For this review, take the finished solid that the model builds, in its own axes (mm). A direction names the side the tool comes from. Give positions to 0.01 mm unless a question says otherwise; leave off trailing zeros. Write each loop counter-clockwise with the first axis right and the second up, starting at its lowest first coordinate (ties: lowest second). Pieces come first, ordered by that corner, then holes.
Q1. Machinability: for faces 1 (the flat face through (1, 30, -11.75)), 2 (the cylindrical face through (0.57, 19.27, -14.4)), 3 (the cylindrical face through (30.43, 43.48, -14.4)), 4 (the flat face through (27, 19, -7)), 5 (the flat face through (13, 37, -1)), which of the approach directions +Z, -Z, +X, -X, +Y, -Y give a long, thin tool a straight path to every point of the face, cutting with its end or side? Answer none if there is none.
Q2. We need section B-B (y = 22.5). Write out the cut boundary in (x, z).
Q3. We need section C-C (x = 13.5). Write out the cut boundary in (y, z), then the cut area to 4 significant figures.
Q4. For line 1 (X direction, y = 22.5, z = -11.2); line 2 (Y direction, x = 13.5, z = -7); line 3 (X direction, y = 7, z = -11.25), list the stretches that pass through material, from the lowest coordinate up.
Q5. Mouldability with a two-part tool opening along X and no side actions: class faces 6 (the flat face through (9.4, 45, -14.3)), 7 (the cylindrical face through (-3.4, 43.48, -0.57)), 8 (the cylindrical face through (26.43, 19.27, -14.4)), 9 (the flat face through (13, 37, -14)) as released by +X, released by -X, zero draft, split by the parting line, or undercut.
Q6. Insertion check: P1, Ø4, axis at x = 4.5, z = -10.5, coming from the +Y side; P2, Ø2, axis at y = 36, z = -6, coming from the -X side; P3, Ø1.5, axis at y = 29.5, z = -10, coming from the -X side; P4, Ø4.5, axis at x = 13.5, y = 22.5, coming from the -Z side. Each pin has a flat end and moves straight along its axis. Give the tip position at first contact, or say it passes through.
Q7. We need section D-D (y = 36.5). Write out the cut boundary in (x, z).
Q8. We need section A-A (z = -6). Give the number of separate pieces and of enclosed holes in the cut face, then the cut area to 3 significant figures.
```python
from build123d import *

# Parameters (mm, degrees)
SKETCH1_W           = 27
SKETCH1_H           = 15
BOSS_EXTRUDE1_DEPTH = 45
SKETCH2_W           = 35
SKETCH2_H           = 15
BOSS_EXTRUDE2_DEPTH = 5
SKETCH3_W           = 23.5
SKETCH3_H           = 13
CUT_EXTRUDE1_DEPTH  = 17
SKETCH4_W           = 8.5
SKETCH4_H           = 3.5
CUT_EXTRUDE2_DEPTH  = 17
SKETCH5_R           = 2.5
CUT_EXTRUDE3_DEPTH  = 17
FILLET1_R           = 2
SKETCH6_R           = 5.75
CUT_EXTRUDE4_DEPTH  = 5


with BuildPart() as part:
    # Sketch1 → Boss-Extrude1 (new body)
    with BuildSketch(Plane(origin=(0, 0, 0), x_dir=(1, 0, 0), z_dir=(0, 1, 0))):
        with Locations((13.5, 7.5)):
            Rectangle(SKETCH1_W, SKETCH1_H)
    extrude(amount=BOSS_EXTRUDE1_DEPTH)

    # Sketch2 → Boss-Extrude2 (add)
    with BuildSketch(Plane(origin=(0, 45, 0), x_dir=(1, 0, 0), z_dir=(0, 1, 0))):
        with Locations((13.5, 7.5)):
            Rectangle(SKETCH2_W, SKETCH2_H)
    extrude(amount=-BOSS_EXTRUDE2_DEPTH)

    # Sketch3 → Cut-Extrude1 (cut)
    with BuildSketch(Plane(origin=(0, 45, 0), x_dir=(1, 0, 0), z_dir=(0, 1, 0))):
        with Locations((13.5, 7.5)):
            Rectangle(SKETCH3_W, SKETCH3_H)
    extrude(amount=-CUT_EXTRUDE1_DEPTH, mode=Mode.SUBTRACT)

    # Sketch4 → Cut-Extrude2 (cut)
    with BuildSketch(Plane.ZY):
        with Locations((-7.5, 29.75)):
            Rectangle(SKETCH4_W, SKETCH4_H)
    extrude(amount=-CUT_EXTRUDE2_DEPTH, mode=Mode.SUBTRACT)

    # Sketch5 → Cut-Extrude3 (cut)
    with BuildSketch(Plane(origin=(0, 0, -15), x_dir=(-1, 0, 0), z_dir=(0, 0, -1))):
        with Locations((-13.5, 22.5)):
            Circle(SKETCH5_R)
    extrude(amount=-CUT_EXTRUDE3_DEPTH, mode=Mode.SUBTRACT)

    # Fillet1
    fillet1_edges = [part.edges().sort_by_distance(p)[0] for p in [
        (0, 40, -7.5),
        (27, 40, -7.5),
    ]]
    fillet(fillet1_edges, radius=FILLET1_R)
    fillet1_2_edges = [part.edges().sort_by_distance(p)[0] for p in [
        (-4, 42.5, -15),
        (-4, 42.5, 0),
        (-4, 40, -7.5),
        (31, 40, -7.5),
        (31, 42.5, 0),
        (31, 42.5, -15),
        (0, 19, -15),
        (0, 19, 0),
        (27, 19, 0),
        (27, 19, -15),
        (27.585786438, 39.414213562, -15),
        (27.585786438, 39.414213562, 0),
        (-0.585786438, 39.414213562, 0),
        (-0.585786438, 39.414213562, -15),
    ]]
    fillet(fillet1_2_edges, radius=FILLET1_R - 0.0001)  # a hair under: the kernel refuses the full size

    # Sketch6 → Cut-Extrude4 (cut)
    with BuildSketch(Plane(origin=(0, 0, -15), x_dir=(-1, 0, 0), z_dir=(0, 0, -1))):
        with Locations((-13.5, 22.5)):
            Circle(SKETCH6_R)
    extrude(amount=-CUT_EXTRUDE4_DEPTH, mode=Mode.SUBTRACT)


solid = part.part
```
Computed:
1. face 1: -X
1. face 2: -Z, -X, -Y
1. face 3: -Z, +X, +Y, -Y
1. face 4: +Z, -Z, +X, -Y
1. face 5: +Y
2. outline: (0, -13) arc R2 ccw to (2, -15) - (7.75, -15) - (7.75, -10) - (11, -10) - (11, 0) - (2, 0) arc R2 ccw to (0, -2) - close; (16, -10) - (19.25, -10) - (19.25, -15) - (25, -15) arc R2 ccw to (27, -13) - (27, -2) arc R2 ccw to (25, 0) - (16, 0) - close
3. outline: (0, -15) - (16.75, -15) - (16.75, -10) - (20, -10) - (20, 0) - (0, 0) - close; (25, -10) - (28, -10) - (28, -1) - (45, -1) - (45, 0) - (25, 0) - close; (28.25, -15) - (45, -15) - (45, -14) - (28.25, -14) - close
3. area: 347.5 mm2
4. line 1: x = 0 to 7.75, 19.25 to 27
4. line 2: y = 0 to 20, 25 to 28
4. line 3: x = 0 to 27
5. face 6: zero draft
5. face 7: released by -X
5. face 8: released by +X
5. face 9: undercut
6. P1: stops at y = 28
6. P2: stops at x = 0
6. P3: stops at x = 25.25
6. P4: passes through
7. outline: (0, -13) arc R2 ccw to (2, -15) - (25, -15) arc R2 ccw to (27, -13) - (27, -2) arc R2 ccw to (25, 0) - (2, 0) arc R2 ccw to (0, -2) - close; hole (1.75, -14) - (25.25, -14) - (25.25, -1) - (1.75, -1) - close
8. separate pieces: 2
8. enclosed holes: 1
8. area: 830 mm2
